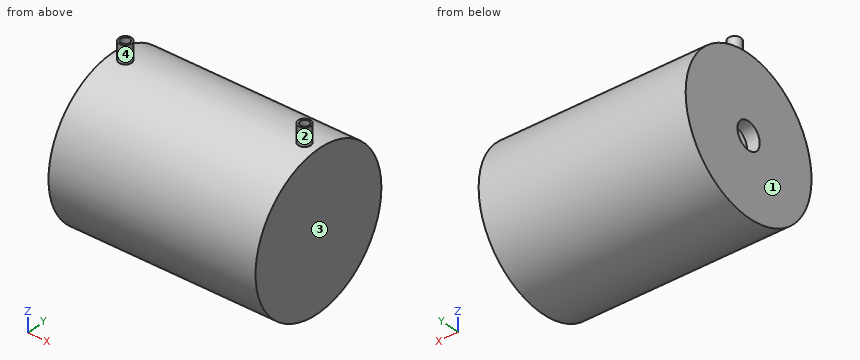
from build123d import *

# Parameters (mm, degrees)
F0_R      = 42.525
F0_R_2    = 40.025
F1_DEPTH  = 50
F2_R      = 42.525
F3_DEPTH  = 7
F6_D      = 15.05
F6_DEPTH  = 12
F6_TIP    = 4.5214761582
F8_R      = 3.5
F9_DEPTH  = 10
F11_D     = 5
F11_DEPTH = 15
F11_TIP   = 1.5021515476


with BuildPart() as f1:
    # F0 (on Right) → F1 (new body, symmetric)
    with BuildSketch(Plane.YZ):
        Circle(F0_R)
        Circle(F0_R_2, mode=Mode.SUBTRACT)
    extrude(amount=F1_DEPTH, both=True)

    # F4: F3 across plane


with BuildPart() as f3:
    # F2 (on face) → F3 (new body)
    with BuildSketch(Plane.YZ.offset(50)):
        Circle(F2_R)
    extrude(amount=F3_DEPTH)


with BuildPart() as f1_1:
    add(f1.part)
    add(f3.part.mirror(Plane.YZ))

    # F6
    with Locations(Plane(origin=(-57, 0, 0), x_dir=(0, -1, 0), z_dir=(-1, 0, 0))):
        with Locations((0, 0)):
            Hole(F6_D / 2, depth=F6_DEPTH)
            with Locations((0, 0, -(F6_DEPTH + F6_TIP / 2))):  # 118° drill point
                Cone(0, F6_D / 2, F6_TIP, mode=Mode.SUBTRACT)


    add(f3.part)  # F9 merges F3
    # F8 (on offset) → F9 (join)
    with BuildSketch(Plane.XY.offset(42.5)):
        with Locations((-49.3345595896, 0)):
            Circle(F8_R)
        with Locations((49.3345595896, 0)):
            Circle(F8_R)
    extrude(amount=F9_DEPTH)

    # F11
    with Locations(Plane.XY.offset(52.5)):
        with Locations((-49.3345595896, 0), (49.3685118854, 0)):
            Hole(F11_D / 2, depth=F11_DEPTH)
            with Locations((0, 0, -(F11_DEPTH + F11_TIP / 2))):  # 118° drill point
                Cone(0, F11_D / 2, F11_TIP, mode=Mode.SUBTRACT)


solid = f1_1.part
Verification items for the finished model (mm, model axes). Face numbers are marked on the shaded views. Give positions to 0.01 mm unless a question says otherwise; leave off trailing zeros. Write each loop counter-clockwise with the first axis right and the second up, starting at its lowest first coordinate (ties: lowest second). Pieces come first, ordered by that corner, then holes.
(1) Gauge pin test, flat ends, axial feed: pin 1 (8 mm diameter, centred on x = -13.5, y = -26.5, fed in from +Z) (3 decimals); pin 2 (6 mm diameter, centred on y = 32, z = -32.5, fed in from -X); pin 3 (4 mm diameter, centred on x = -49.33, y = 0, fed in from +Z); pin 4 (2 mm diameter, centred on x = -48.5, y = 2.5, fed in from -Z). Record the tip position at first contact, or that the pin passes through.
(2) Material ranges on line 1 (Z direction, x = -55.5, y = 0) (3 decimals); line 2 (Z direction, x = -3, y = 0) (3 decimals); line 3 (X direction, y = -8, z = -29.5), recorded low to high.
(3) Cross-section at B-B (z = 0). Enter the section's corners in (x, y) (3 decimals), plus the area to 3 significant figures.
(4) Cross-section at C-C (x = 27). Enter the section's corners in (y, z) (3 decimals).
(5) Cross-section at D-D (z = 34.5). Enter the section's corners in (x, y), plus the area to 3 significant figures.
(6) Cross-section at A-A (y = 0). Enter the section's corners in (x, z) (3 decimals).
(7) Mould release check, pull along X, two halves, no side actions. Record for the marked faces 1, 2, 3 and 4: +X half, -X half, draft (parallel to the pull), parting line (faces both ways), or undercut.
Worked out:
1. pin 1: stops at z = 36.085
1. pin 2: passes through
1. pin 3: stops at z = 37.2
1. pin 4: stops at z = -42.5
2. line 1: z = -42.525 to -7.525, 7.525 to 42.525
2. line 2: z = -42.525 to -40.025, 40.025 to 42.525
2. line 3: x = -57 to -50, 50 to 57
3. outline: (-57, -42.525) - (57, -42.525) - (57, 42.525) - (-57, 42.525) - (-57, 7.525) - (-50, 7.525) - (-50, 40.025) - (50, 40.025) - (50, -40.025) - (-50, -40.025) - (-50, -7.525) - (-57, -7.525) - close
3. area: 1,590 mm2
4. outline: circle Ø85.05 at (0, 0); hole circle Ø80.05 at (0, 0)
5. outline: (-57, -24.86) - (57, -24.86) - (57, 24.86) - (-57, 24.86) - close; hole (-50, -20.29) - (50, -20.29) - (50, 20.29) - (-50, 20.29) - close
5. area: 1,610 mm2
6. outline: (-57, -42.525) - (57, -42.525) - (57, 42.525) - (52.835, 42.525) - (52.835, 52.5) - (51.869, 52.5) - (51.869, 37.5) - (50, 36.377) - (50, -40.025) - (-50, -40.025) - (-50, -7.525) - (-57, -7.525) - close; (-57, 7.525) - (-50, 7.525) - (-50, 36.398) - (-51.835, 37.5) - (-51.835, 52.5) - (-52.835, 52.5) - (-52.835, 42.525) - (-57, 42.525) - close; (-46.835, 40.025) - (46.869, 40.025) - (46.869, 52.5) - (45.835, 52.5) - (45.835, 42.525) - (-45.835, 42.525) - (-45.835, 52.5) - (-46.835, 52.5) - close
7. face 1: -X half
7. face 2: undercut
7. face 3: +X half
7. face 4: undercut
